```python
from build123d import *

# Parameters (mm, degrees)
SKETCH3_R           = 105
SKETCH3_R_2         = 10.2
SKETCH3_R_3         = 9
SKETCH3_R_4         = 3.75
BOSS_EXTRUDE1_DEPTH = 4


with BuildPart() as part:
    # Sketch3 → Boss-Extrude1 (new body)
    with BuildSketch(Plane(origin=(0, 0, 0), x_dir=(1, 0, 0), z_dir=(0, 1, 0))):
        with Locations(Location((0, 0, 0), (0, 0, 270))):
            Circle(SKETCH3_R)
        with Locations(Location((0, 30, 0), (0, 0, 270))):
            Circle(SKETCH3_R_2, mode=Mode.SUBTRACT)
        with Locations(Location((61.871843354, 61.871843354, 0), (0, 0, 270))):
            Circle(SKETCH3_R_3, mode=Mode.SUBTRACT)
        with Locations(Location((0, 87.5, 0), (0, 0, 270))):
            Circle(SKETCH3_R_3, mode=Mode.SUBTRACT)
        with Locations(Location((-61.871843354, 61.871843354, 0), (0, 0, 270))):
            Circle(SKETCH3_R_3, mode=Mode.SUBTRACT)
        with Locations(Location((-87.5, 0, 0), (0, 0, 270))):
            Circle(SKETCH3_R_3, mode=Mode.SUBTRACT)
        with Locations(Location((-61.871843354, -61.871843354, 0), (0, 0, 270))):
            Circle(SKETCH3_R_3, mode=Mode.SUBTRACT)
        with Locations(Location((0, -87.5, 0), (0, 0, 270))):
            Circle(SKETCH3_R_3, mode=Mode.SUBTRACT)
        with Locations(Location((61.871843354, -61.871843354, 0), (0, 0, 270))):
            Circle(SKETCH3_R_3, mode=Mode.SUBTRACT)
        with Locations(Location((87.5, 0, 0), (0, 0, 270))):
            Circle(SKETCH3_R_3, mode=Mode.SUBTRACT)
        with Locations(Location((-21.213203436, -21.213203436, 0), (0, 0, 270))):
            Circle(SKETCH3_R_2, mode=Mode.SUBTRACT)
        with Locations(Location((33.760092737, 13.983888279, 0), (0, 0, 270))):
            Circle(SKETCH3_R_4, mode=Mode.SUBTRACT)
        with Locations(Location((21.213203436, -21.213203436, 0), (0, 0, 270))):
            Circle(SKETCH3_R_2, mode=Mode.SUBTRACT)
    extrude(amount=BOSS_EXTRUDE1_DEPTH)


solid = part.part
```
Could you check a few things on this model? Use its own coordinates, in mm. Give positions to 0.01 mm unless a question says otherwise; leave off trailing zeros. Order: outer loops, then holes, each group sorted by start corner. A loop starts at its lowest first (then second) coordinate and runs counter-clockwise, first axis right, second up.
Q1. We'd pull the mould along X, two halves only. Please class faces 1 (the cylindrical face through (31.326, 1.972, 19.885)), 2 (the cylindrical face through (31.54, 1.97, 100.15)), 3 (the flat face through (1, 4, -1)): +X half, -X half, draft (parallel to the pull), parting line (faces both ways), or undercut.
Q2. Suppose I cut it at D-D, the plane y = 1.5. Count the separate pieces of the cut face and the enclosed holes in it, and give its area (3 significant figures).
Q3. Suppose I cut it at A-A, the plane z = 56. Write out the boundary of the cut face in (x, y), and give its area (3 significant figures).
Q4. Suppose I cut it at C-C, the plane z = 91.5. Write out the boundary of the cut face in (x, y), and give its area (3 significant figures).
Q5. Suppose I cut it at B-B, the plane x = -66.5. Write out the boundary of the cut face in (y, z).
Q6. If I drill on line 1 along X through (y, z) = (1.2, 0.5); line 2 along Z through (x, y) = (-0.5, 3.75); line 3 along X through (y, z) = (1.9, 54), over which ranges is the centre line in solid material (lowest first)?
Q7. I'm going to push flat-ended pins straight in: P1, Ø11, axis at x = 87.5, z = 0, coming from the -Y side; P2, Ø2, axis at y = 2.5, z = -8, coming from the +X side. Where does each tip first touch, or does it pass through?
Solution:
1. face 1: undercut
1. face 2: parting line
1. face 3: draft
2. separate pieces: 1
2. enclosed holes: 12
2. area: 31,600 mm2
3. outline: (-88.82, 0) - (-68.69, 0) - (-68.69, 4) - (-88.82, 4) - close; (-55.05, 0) - (55.05, 0) - (55.05, 4) - (-55.05, 4) - close; (68.69, 0) - (88.82, 0) - (88.82, 4) - (68.69, 4) - close
3. area: 601 mm2
4. outline: (-51.5, 0) - (-8.06, 0) - (-8.06, 4) - (-51.5, 4) - close; (8.06, 0) - (51.5, 0) - (51.5, 4) - (8.06, 4) - close
4. area: 348 mm2
5. outline: (0, -81.26) - (4, -81.26) - (4, -69.59) - (0, -69.59) - close; (0, -54.15) - (4, -54.15) - (4, 54.15) - (0, 54.15) - close; (0, 69.59) - (4, 69.59) - (4, 81.26) - (0, 81.26) - close
6. line 1: x = -105 to -96.49, -78.51 to 78.51, 96.49 to 105
6. line 2: z = -105 to -96.49, -78.51 to -40.19, -19.81 to 78.51, 96.49 to 105
6. line 3: x = -90.05 to -66.23, -57.51 to 57.51, 66.23 to 90.05
7. P1: passes through
7. P2: stops at x = 104.77
